```python
from build123d import *

# Parameters (mm, degrees)
EXTRUDE_1_DEPTH          = 5
EXTRUDE_1_DEPTH_BACK     = 5
SKETCH_1_R               = 4
SKETCH_1_R_2             = 1.5
SKETCH_1_R_3             = 3.999999999999999
SKETCH_1_R_4             = 1.6500000000000021
CUT_EXTRUDE_1_DEPTH      = 2.6
CUT_EXTRUDE_1_DEPTH_BACK = 2.6
SKETCH_2_R               = 10
SKETCH_3_R               = 1.500000000000004
SKETCH_3_R_2             = 1.6500000000000021
EXTRUDE_3_DEPTH          = 10
SKETCH_4_W               = 20.00000000000002
SKETCH_4_H               = 5.2
CUT_EXTRUDE_2_DEPTH      = 10
CHAMFER_1_SIZE           = 0.5


with BuildPart() as part:
    # 草图1 → 凸台-拉伸1 (new, two sides: drawn at the far end of the back side and taken through both)
    # profile 1 of 3: a face of its own
    with BuildSketch(Plane.XY.offset(-EXTRUDE_1_DEPTH_BACK)):
        Circle(SKETCH_1_R)
        Circle(SKETCH_1_R_2, mode=Mode.SUBTRACT)
    # profile 2 of 3: a face of its own
    with BuildSketch(Plane.XY.offset(-EXTRUDE_1_DEPTH_BACK)):
        with BuildLine():
            ThreePointArc((2.241669254584064, 3.3128415224777243), (3.5331768295923327, 1.8752763771860061), (4, 0))
            ThreePointArc((4, -9.8e-16), (1.875276377186004, -3.533176829592334), (-2.241669254584067, -3.312841522477722))
            add(Edge.make_bspline(
                [(-2.2416692545840666, -3.3128415224777275), (4.023288399104954, -7.552091380419048), (17.137885249639094, -10.692937395333647), (31.700941101616845, -7.062033828913657), (37.24166925458407, -3.3128415224777283)],
                knots=[0, 0, 0, 0, 0.5000000000000002, 1, 1, 1, 1], degree=3))
            ThreePointArc((37.24166925458406, -3.312841522477722), (31.687158477522274, -2.2416692545840604), (32.75833074541594, 3.312841522477726))
            add(Edge.make_bspline(
                [(2.2416692545840613, 3.3128415224777203), (2.5417844094553557, 3.1097654287542427), (3.1567145921113204, 2.711097631998411), (4.363329654695279, 1.996321701251651), (5.869996949507693, 1.2242995538785062), (7.677590875082871, 0.4788920232894552), (10.115405251702699, -0.2996699093227729), (13.252057238449053, -0.9025900818361017), (17.317568666800724, -1.0878092080294735), (21.627918427541044, -0.7536952847930135), (25.807284141658094, 0.1095698053821612), (28.992197069652473, 1.2411094397422888), (31.264365551631894, 2.3695049176779595), (32.264190962280374, 2.9784766119300636), (32.75833074541594, 3.312841522477724)],
                knots=[0, 0, 0, 0, 0.03125, 0.0625, 0.125, 0.1875, 0.25, 0.375, 0.5, 0.625, 0.75, 0.875, 0.9375, 1, 1, 1, 1], degree=3))
        make_face()
    # profile 3 of 3: a face of its own
    with BuildSketch(Plane.XY.offset(-EXTRUDE_1_DEPTH_BACK)):
        with Locations((35, 2.24e-15)):
            Circle(SKETCH_1_R_3)
        with Locations((35, 2.24e-15)):
            Circle(SKETCH_1_R_4, mode=Mode.SUBTRACT)
    extrude(amount=EXTRUDE_1_DEPTH + EXTRUDE_1_DEPTH_BACK)

    # 草图2 → 切除-拉伸1 (cut, two sides: drawn at the far end of the back side and taken through both)
    with BuildSketch(Plane.XY.offset(-CUT_EXTRUDE_1_DEPTH_BACK)):
        Circle(SKETCH_2_R)
    extrude(amount=CUT_EXTRUDE_1_DEPTH + CUT_EXTRUDE_1_DEPTH_BACK, mode=Mode.SUBTRACT)

    # 草图3 → 凸台-拉伸3 (add)
    with BuildSketch(Plane(origin=(0, 0, -5), x_dir=(-1, 0, 0), z_dir=(0, 0, -1))):
        with BuildLine():
            Line((-57, 3.9999999999999947), (-35, 4.000000000000001))
            ThreePointArc((-35, 4.000000000000001), (-31.000000000000004, 2.24e-15), (-35, -3.9999999999999956))
            Line((-35, -3.9999999999999956), (-57, -3.9999999999999947))
            ThreePointArc((-57, -3.9999999999999947), (-61, -2.2e-15), (-57, 3.9999999999999947))
        make_face()
        with Locations((-57, -2.69e-15)):
            Circle(SKETCH_3_R, mode=Mode.SUBTRACT)
        with Locations(Location((-35, 2.24e-15, 0), (0, 0, 180))):
            Circle(SKETCH_3_R_2, mode=Mode.SUBTRACT)
    extrude(amount=-EXTRUDE_3_DEPTH)

    # 草图4 → 切除-拉伸2 (cut)
    with BuildSketch(Plane(origin=(1.1e-15, 4.000000000000011, 0), x_dir=(1, -2.8e-16, 0), z_dir=(2.8e-16, 1, 0))):
        with Locations((61.000000000000014, 0)):
            Rectangle(SKETCH_4_W, SKETCH_4_H)
    extrude(amount=-CUT_EXTRUDE_2_DEPTH, mode=Mode.SUBTRACT)

    # 倒角1
    chamfer_1_edges = [part.edges().sort_by_distance(p)[0] for p in [
        (58.50000000000001, -2.51e-15, -5),
        (58.50000000000001, -2.51e-15, 5),
        (33.349999999999994, 1.71e-15, 5),
        (-1.5, 1.8e-16, 5),
        (-1.5, 1.8e-16, -5),
        (33.349999999999994, 1.71e-15, -5),
        (17.466337621201156, -0.999163570519443, 5),
        (-3.3128415224777235, 2.2416692545840653, 5),
        (17.466337621201156, -0.999163570519443, 5),
        (46.58588320296925, -3.999999999999995, 5),
        (46.58588320296925, -3.999999999999995, -5),
        (33.82768734757124, 3.824353938243094, 5),
        (61, -2e-17, -5),
        (61, -2e-17, 5),
        (46, 3.999999999999998, -5),
        (46, 3.999999999999998, 5),
        (17.466337621201156, -0.999163570519443, -5),
        (-3.3128415224777235, 2.2416692545840653, -5),
        (33.82768734757124, 3.8243539382430947, -5),
        (17.466337621201156, -0.999163570519443, -5),
    ]]
    chamfer(chamfer_1_edges, length=CHAMFER_1_SIZE)


solid = part.part
```
Input: part model. Units: mm. Frame: model coordinates. A direction names the side the tool comes from. Round coordinates to 2 decimals unless told otherwise and drop trailing zeros. Loops run counter-clockwise (first coordinate to the right, second up) from the corner with the lowest first, then second, coordinate; pieces in that order, holes last. Notation, with made-up numbers: (21, -29.75) - (29, -29.75) arc R26 cw to (29, -12.75) - close; hole circle Ø5 at (57.25, 11.5). An arc over 180 degrees is marked (long way). One line per item, written item: value. Start each with the question number.
(1) Draft query along Z for faces 1 (the conical face through (60.64, -0.08, -4.86)), 2 (the flat face through (3, -2, 2.6)), 3 (the cylindrical face through (-3.263, 2.314, -3.563)). Return one class per face: +Z half, -Z half, draft (parallel to the pull), parting line (faces both ways), or undercut.
(2) Contact query for flat-ended pins moving along their axis: P1, Ø1, axis at x = 28, z = -4, coming from the -Y side; P2, Ø3.5, axis at x = 57, y = 0, coming from the -Z side; P3, Ø5, axis at x = 57, y = 0, coming from the +Z side; P4, Ø6, axis at x = 43, z = 0.5, coming from the -Y side. Output: stop coordinate, or through.
(3) Section B-B, the plane x = 0. Count the separate pieces of the cut face and the enclosed holes in it, plus the area to 3 significant figures.
(4) Ray query, line 1 (Z direction, x = 51.5, y = 0.25); line 2 (Y direction, x = 57, z = -3); line 3 (Y direction, x = 44, z = -1). Return the intervals inside material, ascending. Write a range as [from, to].
(5) Access query for faces 4 (the conical face through (33.88, 3.58, 4.75)), 5 (the flat face through (3, -2, -2.6)), 6 (the flat face through (55, 0, -2.6)), 7 (the cylindrical face through (33.84, 3.83, -0.06)). Directions: +Z, -Z, +X, -X, +Y, -Y. A direction counts if a zero-diameter tool reaches every point of the face in a straight line with its end or side. Return the directions, or none.
(6) Section A-A, the plane x = 38.5. Return loops of the section in (y, z).
Results below:
1. face 1: -Z half
1. face 2: undercut
1. face 3: draft
2. P1: y = -7.62
2. P2: z = -4.75
2. P3: z = 5
2. P4: y = -4
3. separate pieces: 4
3. enclosed holes: 0
3. area: 26.4 mm^2
4. line 1: [-5, -2.6], [2.6, 5]
4. line 2: [-4, -1.5], [1.5, 4]
4. line 3: [-4, 4]
5. face 4: +Z, +Y
5. face 5: -X, +Y
5. face 6: +X, +Y, -Y
5. face 7: +Z, -Z, +Y
6. outline: (-4, -4.5) - (-3.5, -5) - (3.5, -5) - (4, -4.5) - (4, 4.5) - (3.5, 5) - (-3.5, 5) - (-4, 4.5) - close
